Geometry: final body of the model. Coordinates: model frame, mm. A direction names the side the tool comes from. Round coordinates to 2 decimals unless told otherwise and drop trailing zeros. Put each result on its own line as item: value. Start each with the question number.
1) Material intervals for probe 1 along X at (y, z) = (1.45, 720.5); probe 2 along Z at (x, y) = (-180, 0.25); probe 3 along Z at (x, y) = (-158, 0.6), sorted ascending. Write a range as [from, to].
2) First-contact query: P1, Ø1.8, axis at x = -143.51, z = 687.9, coming from the +Y side; P2, Ø15.5, axis at x = -272.58, z = 730.31, coming from the -Y side; P3, Ø0.5, axis at x = -145, y = 1, coming from the -Z side; P4, Ø0.5, axis at x = -311.5, y = 0.5, coming from the +Z side. Flat tips, straight axial feed; report the tip coordinate or a pass-through.
3) Draft query along X for faces 1 (the flat face through (-296.89, 0.75, 618.49)), 2 (the flat face through (-225, 0, 675)), 3 (the flat face through (-172.26, 0.751, 735.937)), 4 (the flat face through (-175.617, 0.751, 748.615)). Return one class per face: pulls with the +X half, pulls with the -X half, needs draft (parallel to the pull), parting line crosses it, or undercut.
4) Access query for faces 5 (the flat face through (-292.32, 0.75, 733.78)), 6 (the flat face through (-179.29, 0.75, 596.12)), 7 (the flat face through (-279.541, 0.751, 737.494)), 8 (the flat face through (-280.59, 0.75, 602.26)). Directions: +Z, -Z, +X, -X, +Y, -Y. A direction counts if a zero-diameter tool reaches every point of the face in a straight line with its end or side. Return the directions, or none.
5) Section A-A, the plane y = 0.55. Count the separate pieces of the cut face and the enclosed holes in it, then the cut area to 3 significant figures.
Autodesk Inventor part; units mm, degrees
ref_plane "YZ Plane" through (0, 0, 0) normal (1, 0, 0) x (0, 1, 0)
ref_plane "XZ Plane" through (0, 0, 0) normal (0, 1, 0) x (-1, 0, 0)
ref_plane "XY Plane" through (0, 0, 0) normal (0, 0, 1) x (1, 0, 0)
sketch "Sketch1" plane through (0, 0, 0) normal (0, 1, 0) x (-1, 0, 0)
  line L0 (248.9211, 774.0716) -> (204.4366, 774.0716)
  line L1 (204.4366, 574.0727) -> (249.4778, 574.0727)
  line L2 (316.3476, 688.3671) -> (303.3476, 688.3671)
  line L3 (303.3476, 688.3671) -> (303.3476, 665.3671)
  line L4 (303.3476, 665.3671) -> (316.3476, 665.3671)
  line L5 (137.0102, 685.5727) -> (150.0102, 685.5727)
  line L6 (150.0102, 685.5727) -> (150.0102, 662.5836)
  line L7 (150.0102, 662.5836) -> (137.0102, 662.5836)
  line L8 (316.3476, 641.3894) -> (316.3476, 665.3671)
  line L9 (316.3476, 688.3671) -> (316.3476, 706.6452)
  line L10 (137.0102, 706.6452) -> (137.0102, 685.5727)
  line L11 (137.0102, 662.5836) -> (137.0102, 641.4992)
  line L12 (280.7152, 754.704) -> (271.5228, 745.5116)
  line L13 (271.5228, 745.5116) -> (287.7863, 729.2481)
  line L14 (287.7863, 729.2481) -> (296.9787, 738.4405)
  line L15 (158.3637, 607.7192) -> (167.5561, 616.9116)
  line L16 (167.5561, 616.9116) -> (183.8196, 600.6481)
  line L17 (183.8196, 600.6481) -> (174.6272, 591.4557)
  line L18 (145.7969, 620.2859) -> (158.3637, 607.7192)
  line L19 (174.6272, 591.4557) -> (183.2234, 582.8595)
  line L20 (307.5608, 727.8584) -> (296.9787, 738.4405)
  line L21 (280.7152, 754.704) -> (270.1344, 765.2849)
  line L22 (171.0855, 753.147) -> (180.2779, 743.9546)
  line L23 (180.2779, 743.9546) -> (164.0144, 727.6911)
  line L24 (164.0144, 727.6911) -> (154.822, 736.8835)
  line L25 (301.4465, 613.9871) -> (292.1989, 623.1239)
  line L26 (292.1989, 623.1239) -> (276.0337, 606.7628)
  line L27 (276.0337, 606.7628) -> (285.2813, 597.626)
  line L28 (270.8184, 582.9877) -> (285.2813, 597.626)
  line L29 (301.4465, 613.9871) -> (307.6882, 620.3044)
  line L30 (183.2234, 765.2849) -> (171.0855, 753.147)
  line L31 (154.822, 736.8835) -> (145.7969, 727.8584)
  arc A0 (261.9333, 773.4859) -> (260.5191, 774.0716) centre (260.5191, 772.0716) ccw
  arc A1 (270.1344, 765.2849) -> (248.9211, 774.0716) centre (248.9211, 744.0716) ccw
  arc A2 (204.4366, 774.0716) -> (183.2234, 765.2849) centre (204.4366, 744.0716) ccw
  arc A3 (145.7969, 727.8584) -> (137.0102, 706.6452) centre (167.0102, 706.6452) ccw
  arc A4 (137.0102, 641.4992) -> (145.7969, 620.2859) centre (167.0102, 641.4992) ccw
  arc A5 (183.2234, 582.8595) -> (204.4366, 574.0727) centre (204.4366, 604.0727) ccw
  arc A6 (249.4778, 574.0727) -> (270.8184, 582.9877) centre (249.4778, 604.0727) ccw
  arc A7 (307.6882, 620.3044) -> (316.3476, 641.3894) centre (286.3476, 641.3894) ccw
  arc A8 (316.3476, 706.6452) -> (307.5608, 727.8584) centre (286.3476, 706.6452) ccw
  circle A9 centre (279.0199, 600.5369) radius 1.5
  circle A10 centre (309.8476, 663.0421) radius 1.5
  circle A11 centre (309.8476, 690.6921) radius 1.5
  circle A12 centre (294.03, 732.1968) radius 1.5
  circle A13 centre (274.4715, 751.7554) radius 1.5
  circle A14 centre (157.7707, 730.6398) radius 1.5
  circle A15 centre (143.5102, 687.9027) radius 1.5
  circle A16 centre (143.5102, 660.2536) radius 1.5
  circle A17 centre (161.3124, 613.9629) radius 1.5
  circle A18 centre (177.3292, 750.1983) radius 1.5
  circle A19 centre (180.5174, 594.0508) radius 1.5
  circle A20 centre (298.4603, 620.213) radius 1.5
  circle A21 centre (263.158, 720.311) radius 1.25
  circle A22 centre (187.658, 720.311) radius 1.25
  circle A23 centre (263.158, 664.811) radius 1.25
  circle A24 centre (187.658, 664.811) radius 1.25
  line L32 (263.158, 720.311) -> (187.658, 720.311)
  line L33 (263.158, 664.811) -> (187.658, 664.811)
  line L34 (263.158, 720.311) -> (263.158, 664.811)
  line L35 (187.658, 720.311) -> (187.658, 664.811)
  circle A25 centre (256.4035, 659.5938) radius 1.25
  circle A26 centre (199.9035, 659.5938) radius 1.25
  circle A27 centre (256.4035, 623.0938) radius 1.25
  circle A28 centre (199.9035, 623.0938) radius 1.25
  line L36 (256.4035, 659.5938) -> (199.9035, 659.5938)
  line L37 (256.4035, 659.5938) -> (256.4035, 623.0938)
  line L38 (256.4035, 623.0938) -> (199.9035, 623.0938)
  line L39 (199.9035, 623.0938) -> (199.9035, 659.5938)
  circle A29 centre (179.2172, 728.7518) radius 6
  circle A30 centre (160.0102, 674.0836) radius 6
  circle A31 centre (182.7589, 615.8509) radius 6
  circle A32 centre (277.0028, 621.9717) radius 6
  circle A33 centre (294.03, 676.8671) radius 6
  circle A34 centre (272.5835, 730.3088) radius 6
  point P0 (0, 0)
  point P1 (316.3476, 774.0716)
  point P2 (137.0102, 574.0727)
  point P3 (137.0102, 774.0716)
  point P4 (317.0102, 574.0727)
  point P5 (262.0102, 574.0727)
  point P6 (316.3476, 629.0688)
  point P7 (316.3476, 719.0716)
  point P8 (261.3476, 774.0716)
  point P9 (192.0102, 774.0716)
  point P10 (137.0102, 719.0716)
  point P11 (137.0102, 629.0727)
  point P12 (192.0102, 574.0727)
  dimension "d0" = 200
  dimension "d1" = 180
  dimension "d2" = 55
  dimension "d3" = 55
  dimension "d4" = 55
  dimension "d5" = 55
  dimension "d6" = 55
  dimension "d7" = 55
  dimension "d8" = 55
  dimension "d9" = 55
  dimension "d10" = 13
  dimension "d11" = 23
  dimension "d13" = 13
  dimension "d14" = 13
  dimension "d15" = 23
  dimension "d18" = 77.7818
  dimension "d21" = 13
  dimension "d24" = 23
  dimension "d26" = 23
  dimension "d30" = 23
  dimension "d32" = 2
  dimension "d33" = 30
  dimension "d36" = 3
  dimension "d38" = 3
  dimension "d39" = 3
  dimension "d40" = 3
  dimension "d41" = 3
  dimension "d43" = 3
  dimension "d44" = 3
  dimension "d45" = 3
  dimension "d46" = 3
  dimension "d49" = 6.5
  dimension "d50" = 2.325
  dimension "d53" = 2.325
  dimension "d54" = 6.5
  dimension "d55" = 2.33
  dimension "d56" = 6.5
  dimension "d57" = 2.33
  dimension "d58" = 6.5
  dimension "d60" = 3
  dimension "d61" = 6.5
  dimension "d62" = 2.33
  dimension "d63" = 2.33
  dimension "d64" = 6.5
  dimension "d65" = 6.5
  dimension "d66" = 2.33
  dimension "d67" = 6.5
  dimension "d68" = 2.33
  dimension "d69" = 2.33
  dimension "d70" = 6.5
  dimension "d71" = 13
  dimension "d72" = 6
  dimension "d73" = 2.33
  dimension "d74" = 3
  dimension "d75" = 13
  dimension "d78" = 2.33
  dimension "d79" = 6.5
  dimension "d80" = 3
  dimension "d81" = 6.5
  dimension "d82" = 2.33
  dimension "d85" = 9.2476
  dimension "d86" = 13
  dimension "d87" = 13
  dimension "d88" = 13
extrude "Extrusion1" add sketch "Sketch1" along normal blind 1.524 contours A1 L21 L12 L13 L14 L20 A8 L9 L2 L3 L4 L8 A7 L29 L25 L26 L27 L28 A6 L1 A5 L19 L17 L16 L15 L18 A4 L11 L7 L6 L5 L10 A3 L31 L24 L23 L22 L30 A2 L0 | A9 | A10 | A11 | A12 | A13 | A14 | A15 | A16 | A17 | A18 | A19 | A20 | A21 L34 L32 | L32 L34 A21 | A21 L34 A23 L33 A24 L35 A22 L32 | L32 L35 A22 | A22 L35 L32 | L34 L33 A23 | A23 L33 L34 | L35 L33 A24 | A24 L33 L35 | A25 L37 L36 | L36 L37 A25 | A25 L37 A27 L38 A28 L39 A26 L36 | L36 L39 A26 | A26 L39 L36 | L37 L38 A27 | A27 L38 L37 | L39 L38 A28 | A28 L38 L39 | A29 | A30 | A31 | A32 | A33 | A34
extrude "Extrusion2" cut sketch "Sketch1" along normal blind 200 contours A9 | A10 | A11 | A12 | A13 | A14 | A15 | A16 | A17 | A18 | A19 | A20
extrude "Extrusion3" cut sketch "Sketch1" along normal blind 200 contours A29 | A30 | A31 | A32 | A33 | A34
extrude "Extrusion5" cut sketch "Sketch1" along normal blind 200 contours A21 L34 L32 | L32 L34 A21 | L32 L35 A22 | A22 L35 L32 | L34 L33 A23 | A23 L33 L34 | L35 L33 A24 | A24 L33 L35 | A25 L37 L36 | L36 L37 A25 | L36 L39 A26 | A26 L39 L36 | L37 L38 A27 | A27 L38 L37 | L39 L38 A28 | A28 L38 L39
properties part number "Base"
Result sheet:
1. probe 1: x = [-312.96, -264.39], [-261.92, -188.89], [-186.42, -140.4]
1. probe 2: z = [586.08, 592.64], [595.46, 596.83], [604.47, 610.52], [621.18, 722.8], [734.7, 743.68], [744.23, 762.06]
1. probe 3: z = [608.08, 668.43], [679.74, 729.16], [732.12, 733.71]
2. P1: passes through
2. P2: stops at y = 0
2. P3: stops at z = 620.85
2. P4: stops at z = 723.37
3. face 1: undercut
3. face 2: needs draft
3. face 3: undercut
3. face 4: pulls with the +X half
4. face 5: +Z, +Y, -Y
4. face 6: +X, +Y, -Y
4. face 7: +Y, -Y
4. face 8: -X, +Y, -Y
5. separate pieces: 1
5. enclosed holes: 26
5. area: 27,100 mm2
